The model under review builds one solid part; all positions refer to its coordinate system, in mm. A direction names the side the tool comes from. Coordinates: 2 decimals unless noted, no trailing zeros. Loops run counter-clockwise (first coordinate to the right, second up) from the corner with the lowest first, then second, coordinate; pieces in that order, holes last. Notation, with made-up numbers: M 56.25,73 L 110.25,73 A10 ccw 110.25,77 Z; hole C 10,24 d9. An arc over 180 degrees is marked long. Use CSV: the item, a comma, the result in double quotes. Start each with the question number.
1. Add section C-C, the plane z = 10. State how many separate pieces and enclosed holes the cut face has, then the cut area to 3 significant figures.
2. For L1, parallel to Y at x = 0, z = 4.35; L2, parallel to Z at x = -34.5, y = 27.5; L3, parallel to X at y = 26, z = 16.75, list the stretches that pass through material, from the lowest coordinate up.
3. Add section D-D, the plane x = -38. Write out the cut boundary in (y, z).
4. Draft analysis for pull direction Z (two halves, no side actions). For faces 1 (the cylindrical face through (27.76, 32.25, 8.96)), 2 (the cylindrical face through (-28, -21, 15)), 3 (the flat face through (23.1, -26.5, 0)), 4 (the cylindrical face through (-13.527, 36.203, 8.958)), state which applies: +Z half, -Z half, draft (parallel to the pull), parting line (faces both ways), or undercut.
5. Tool access review of faces 5 (the cylindrical face through (20.765, -39.923, 14.958)), 6 (the flat face through (23.1, -26.5, 12)): name each direction out of +Z, -Z, +X, -X, +Y, -Y from which nothing blocks a thin tool from reaching the whole face with its end or side.
6. Add section A-A, the plane y = 0. Write out the cut boundary in (x, z).
7. Clearance check with flat-ended pins moving along their axes: P1, Ø3, axis at x = 18, z = 6, coming from the -Y side; P2, Ø2, axis at y = 32.5, z = 4.5, coming from the +X side; P3, Ø10, axis at x = -34, y = -23, coming from the -Z side; P4, Ø6, axis at x = 22, z = 13, coming from the +Y side. State where each tip first meets the part, or that it passes through.
from build123d import *

# Parameters (mm, degrees)
SKETCH_R      = 45
SKETCH_R_2    = 35
PAD_DEPTH     = 6
SKETCH002_R   = 4
PAD001_DEPTH  = 6
SKETCH003_R   = 45
SKETCH003_R_2 = 35
PAD002_DEPTH  = 6


with BuildPart() as part:
    # Sketch → Pad (new body)
    with BuildSketch(Plane.XY):
        Circle(SKETCH_R)
        Circle(SKETCH_R_2, mode=Mode.SUBTRACT)
    extrude(amount=PAD_DEPTH)

    # Sketch002 (on Face4 of Pad) → Pad001 (join)
    with BuildSketch(Plane.XY.offset(6)):
        with Locations((10.352762, 38.637033)):
            Circle(SKETCH002_R)
        with Locations((28.284271, 28.284271)):
            Circle(SKETCH002_R)
        with Locations((38.637033, 10.352762)):
            Circle(SKETCH002_R)
        with Locations((38.637033, -10.352762)):
            Circle(SKETCH002_R)
        with Locations((28.284271, -28.284271)):
            Circle(SKETCH002_R)
        with Locations((10.352762, -38.637033)):
            Circle(SKETCH002_R)
        with Locations((-10.352762, -38.637033)):
            Circle(SKETCH002_R)
        with Locations((-28.284271, -28.284271)):
            Circle(SKETCH002_R)
        with Locations((-38.637033, -10.352762)):
            Circle(SKETCH002_R)
        with Locations((-38.637033, 10.352762)):
            Circle(SKETCH002_R)
        with Locations((-28.284271, 28.284271)):
            Circle(SKETCH002_R)
        with Locations((-10.352762, 38.637033)):
            Circle(SKETCH002_R)
    extrude(amount=PAD001_DEPTH)

    # Sketch003 (on Face19 of Pad001) → Pad002 (join)
    with BuildSketch(Plane.XY.offset(12)):
        Circle(SKETCH003_R)
        Circle(SKETCH003_R_2, mode=Mode.SUBTRACT)
    extrude(amount=PAD002_DEPTH)


solid = part.part
Computed:
1,separate pieces,"12"
1,enclosed holes,"0"
1,area,"603 mm^2"
2,L1,"y = -45 to -35, 35 to 45"
2,L2,"z = 0 to 6, 12 to 18"
2,L3,"x = -36.73 to -23.43, 23.43 to 36.73"
3,outline,"M -24.1,0 L 24.1,0 L 24.1,6 L 14.3,6 L 14.3,12 L 24.1,12 L 24.1,18 L -24.1,18 L -24.1,12 L -14.3,12 L -14.3,6 L -24.1,6 Z; hole M -6.4,6 L 6.4,6 L 6.4,12 L -6.4,12 Z"
4,face 1,"undercut"
4,face 2,"draft"
4,face 3,"-Z half"
4,face 4,"undercut"
5,face 5,"+Z, -Z"
5,face 6,"none"
6,outline,"M -45,0 L -35,0 L -35,6 L -45,6 Z; M -45,12 L -35,12 L -35,18 L -45,18 Z; M 35,0 L 45,0 L 45,6 L 35,6 Z; M 35,12 L 45,12 L 45,18 L 35,18 Z"
7,P1,"stops at y = -41.87"
7,P2,"stops at x = 32.14"
7,P3,"stops at z = 0"
7,P4,"stops at y = 40.79"
